Geometry check sheet. Reference: the model listing, model coordinates, mm. A direction names the side the tool comes from. Coordinates: 2 decimals unless noted, no trailing zeros. Write each loop counter-clockwise with the first axis right and the second up, starting at its lowest first coordinate (ties: lowest second). Pieces come first, ordered by that corner, then holes.
from build123d import *

# Parameters (mm, degrees)
F0_W     = 200
F0_H     = 200
F1_DEPTH = 100
F2_R     = 90
F3_DEPTH = 25
F4_R     = 70
F5_DEPTH = 25


with BuildPart() as f1:
    # F0 (on Front) → F1 (new body, symmetric)
    with BuildSketch(Plane.XZ):
        Rectangle(F0_W, F0_H)
    extrude(amount=F1_DEPTH, both=True)

    # F2 (on face) → F3 (cut)
    with BuildSketch(Plane.XY.offset(100)):
        Circle(F2_R)
    extrude(amount=-F3_DEPTH, mode=Mode.SUBTRACT)

    # F4 (on face) → F5 (cut)
    with BuildSketch(Plane.XY.offset(75)):
        Circle(F4_R)
    extrude(amount=-F5_DEPTH, mode=Mode.SUBTRACT)


solid = f1.part
1. Sectioned sample at D-D, the plane x = -79.5. Record the boundary of the cut face in (y, z), and give its area (3 significant figures).
Computed values:
outline: (-100, -100) - (100, -100) - (100, 100) - (42.19, 100) - (42.19, 75) - (-42.19, 75) - (-42.19, 100) - (-100, 100) - close
area: 37,900 mm2
2. Gauge pin test, flat end, axial feed: pin 1 Ø4 at (x, y) = (-23.5, -50.5) entering from +Z. Record the tip position at first contact, or that the pin passes through.
Computed values:
pin 1: stops at z = 50
3. Draft check along X on faces 1 (the flat face through (-90.3, -1.4, 100)), 2 (the cylindrical face through (41.53, -79.845, 87.675)), 3 (the flat face through (-100, -1, -1)). Enter one of: released by +X, released by -X, zero draft, split by the parting line, or undercut.
Computed values:
face 1: zero draft
face 2: undercut
face 3: released by -X
4. Sectioned sample at A-A, the plane z = 88.5. Record the boundary of the cut face in (x, y), and give its area (3 significant figures).
Computed values:
outline: (-100, -100) - (100, -100) - (100, 100) - (-100, 100) - close; hole circle Ø180 at (0, 0)
area: 14,600 mm2
5. Access from +Z, -Z, +X, -X, +Y, -Y to the whole of each face (thin tool, end or side, straight path). Record for faces 4 (the flat face through (100, -1, -1)), 5 (the cylindrical face through (-55.55, -42.594, 62.675)).
Computed values:
face 4: +Z, -Z, +X, +Y, -Y
face 5: +Z
6. Sectioned sample at B-B, the plane x = 0. Record the boundary of the cut face in (y, z).
Computed values:
outline: (-100, -100) - (100, -100) - (100, 100) - (90, 100) - (90, 75) - (70, 75) - (70, 50) - (-70, 50) - (-70, 75) - (-90, 75) - (-90, 100) - (-100, 100) - close
7. Thickness scan on line 1 along Y through (x, z) = (0, 70); line 2 along Y through (x, z) = (0, 94.5); line 3 along Z through (x, y) = (-47, 0.5). Record the ranges inside material, lowest first.
Computed values:
line 1: y = -100 to -70, 70 to 100
line 2: y = -100 to -90, 90 to 100
line 3: z = -100 to 50
